Can you work these out from the model? Positions are in its coordinate system, mm. Give positions to 0.01 mm unless a question says otherwise; leave off trailing zeros. Loops run counter-clockwise (first coordinate to the right, second up) from the corner with the lowest first, then second, coordinate; pieces in that order, holes last. Notation, with made-up numbers: (47, 25.25) - (90, 25.25) arc R22 cw to (90, 35.25) - close; hole circle Ø1 at (89.25, -35). An arc over 180 degrees is marked (long way). Answer in a Markdown table with one row per item.
Autodesk Inventor part; units mm, degrees
ref_plane "Work Plane2" through (0, -32.5, -80) normal (0, 0, -1) x (0, 1, 0)
ref_plane "Work Plane1" through (0, 0, 27.5) normal (0, 0, 1) x (1, 0, 0)
ref_plane "Work Plane3" through (0, 0, -200) normal (0, 0, -1) x (-1, 0, 0)
sketch "Sketch6" plane through (0, 0, 0) normal (1, 0, 0) x (0, 1, 0)
  circle A0 centre (0, 0) radius 32.5
  line L0 (-32.5, 0) -> (-32.5, -80)
  line L1 (-32.5, -80) -> (32.5, -80)
  line L2 (32.5, -80) -> (32.5, 0)
  line L3 (0, 0) -> (0, -80) construction
  line L4 (-32.5, -60) -> (32.5, -60)
  circle A1 centre (0, 0) radius 40
  point P0 (32.5, -23.3184)
  point P1 (23.3184, -32.5)
  point P2 (0, -40)
  point P3 (-32.5, -23.3184)
  dimension "d38" = 65
  dimension "d39" = 80
  dimension "d74" = 80
  dimension "d75" = 20
extrude "Extrusion8" add sketch "Sketch6" along normal mid plane 55 contours L2 L4 L0 A1
ref_plane "Work Plane2" through (0, -32.5, -80) normal (0, 0, -1) x (0, 1, 0)
ref_plane "Work Plane1" through (0, 0, 27.5) normal (0, 0, 1) x (1, 0, 0)
sketch "Sketch3" plane through (0, -32.5, -80) normal (0, 0, -1) x (0, 1, 0)
  circle A0 centre (32.5, 0) radius 27.5
  line L0 (65, -27.5) -> (65, 27.5)
  circle A1 centre (32.5, 0) radius 37.5
  dimension "d48" = 10
  dimension "d73" = 55
loft "Loft1" add profiles "Sketch3" section 1 edges at (0, 32.5, -60) (27.5, 0, -60) (0, -32.5, -60) (-27.5, 0, -60) contours A0
sketch "Sketch7" plane through (0, 0, 0) normal (1, 0, 0) x (0, 1, 0)
  line L0 (20.9931, -80) -> (-20.9931, -80)
  line L1 (0, -80) -> (0, -200)
  point P0 (0, 0)
  dimension "d52" = 120
ref_plane "Work Plane3" through (0, 0, -200) normal (0, 0, -1) x (-1, 0, 0)
extrude "Extrusion1" add sketch "Sketch3" along normal blind 100 contours A0
sketch "Sketch5" plane through (0, 0, -180) normal (0, 0, -1) x (-1, 0, 0)
  circle A0 centre (0, 0) radius 10
  point P0 (0, 0)
  dimension "d35" = 20
extrude "Extrusion7" [suppressed]
fillet "Fillet6" radius 10 2 edges at (0, -32.5, -23.3184) (0, 32.5, -23.3184)
properties part number "shank_2"
Q1. If I drill on line 1 (Z direction, x = -8, y = -7.5); line 2 (Z direction, x = 5.5, y = 25.5); line 3 (X direction, y = -17, z = -106), over which ranges is the centre line in solid material (lowest first)? Write a range as [from, to].
Checked values:
| item | result |
|---|---|
| line 1 | z = [-180, -39.29] |
| line 2 | z = [-180, -35.11] |
| line 3 | x = [-21.62, 21.62] |
Q2. If we mould it in two halves opening along Y, with no side actions, what happens to faces 1 (the face through (0, 0, -40)), 2 (the face through (0, -32.5, -52)), 3 (the face through (26.846, -5.961, -129.3)), 4 (the face through (-27.5, 0, -50))? For each: released by +Y, released by -Y, zero draft, split by the parting line, or undercut.
Checked values:
| item | result |
|---|---|
| face 1 | undercut |
| face 2 | released by -Y |
| face 3 | split by the parting line |
| face 4 | zero draft |
Q3. For pin 1 (1 mm diameter, centred on x = -15, y = -26, fed in from -Z); pin 2 (2 mm diameter, centred on y = -17, z = -128.5, fed in from +X); pin 3 (8 mm diameter, centred on y = 13.5, z = -69, fed in from +X), each with a flat end and sliding along its axis, tell me the tip position at first contact or that it passes through.
Checked values:
| item | result |
|---|---|
| pin 1 | stops at z = -76.24 |
| pin 2 | stops at x = 22.37 |
| pin 3 | stops at x = 27.09 |
Q4. Imagine slicing it at A-A, the plane z = -156. Write out the boundary of the cut face in (x, y), and give its area (3 significant figures).
Checked values:
| item | result |
|---|---|
| outline | circle Ø55 at (0, 0) |
| area | 2,380 mm² |
